Verification items for the finished model (mm, model axes). A direction names the side the tool comes from. Round coordinates to 2 decimals unless told otherwise and drop trailing zeros. Order: outer loops, then holes, each group sorted by start corner. A loop starts at its lowest first (then second) coordinate and runs counter-clockwise, first axis right, second up. Notation, with made-up numbers: M 88,-25.5 L 105,-25.5 A22 ccw 105,-4.5 Z; hole C 13.5,75.5 d10. An arc over 180 degrees is marked long. Use CSV: the item, a comma, the result in double quotes. Start each with the question number.
Q1. Sectioned sample at A-A (y = 5.1). Enter the section's corners in (x, z), and give its area (3 significant figures).
Q2. Sectioned sample at B-B (x = 8). Enter the section's corners in (y, z), and give its area (3 significant figures).
Q3. Sectioned sample at D-D (x = 61.5). Enter the section's corners in (y, z).
Q4. Gauge pin test, flat ends, axial feed: pin 1 Ø4.5 at (x, y) = (27.53, -2.9) entering from +Z; pin 2 Ø8.5 at (x, z) = (10.5, 11) entering from +Y; pin 3 Ø6 at (x, y) = (83.63, -2.9) entering from +Z; pin 4 Ø5 at (y, z) = (-3, -7) entering from -X. Record the tip position at first contact, or that the pin passes through.
Q5. Sectioned sample at C-C (y = -38.9). State how many separate pieces and enclosed holes the cut face has, and give its area (3 significant figures).
Q6. Scan lines: line 1 (X direction, y = 5, z = -23); line 2 (Y direction, x = 97.5, z = 2.5); line 3 (Z direction, x = 101.5, y = -38.9). Record each from-to range of solid material in increasing order.
Q7. Mould release check, pull along X, two halves, no side actions. Record for faces 1 (the face through (85.735, -40.244, -22.486)), 2 (the face through (0, 0, -23)), 3 (the face through (55, -42, 23.5)): +X half, -X half, draft (parallel to the pull), parting line (faces both ways), or undercut.
Q8. Set-up check for faces 4 (the face through (7.4, -27.86, 0.33)), 5 (the face through (8, -23.2, 1)), 6 (the face through (61, 41.5, 1)), 7 (the face through (100.99, -36.43, 9.46)): record each of +Z, -Z, +X, -X, +Y, -Y from which the full face is reachable in a straight line by a thin tool's end or side.
```python
from build123d import *

# Parameters (mm, degrees)
PAD_DEPTH       = 15
SKETCH001_W     = 87
SKETCH001_H     = 47
SKETCH003_W     = 87
SKETCH003_H     = 47
PAD001_DEPTH    = 82
POCKET_DEPTH    = 45
SKETCH009_R     = 2.5
POCKET001_DEPTH = 5
SKETCH010_R     = 2.5
POCKET002_DEPTH = 5


with BuildPart() as part:
    # Sketch → Pad (new body)
    with BuildSketch(Plane.YZ):
        with BuildLine():
            Line((-25.2, 23.5), (25.2, 23.5))
            ThreePointArc((25.2, -23.5), (27.86, 0), (25.2, 23.5))
            Line((25.2, -23.5), (-25.2, -23.5))
            ThreePointArc((-25.2, 23.5), (-27.86, 0), (-25.2, -23.5))
        make_face()
    extrude(amount=PAD_DEPTH)

    # Sketch002 (on Face6 of Pad) → AdditiveLoft section 0
    with BuildSketch(Plane.YZ.offset(15)):
        with BuildLine():
            Line((-25.2, 23.5), (25.2, 23.5))
            ThreePointArc((25.2, -23.5), (27.86, 0), (25.2, 23.5))
            Line((-25.2, -23.5), (25.2, -23.5))
            ThreePointArc((-25.2, 23.5), (-27.86, 0), (-25.2, -23.5))
        make_face()
    # Sketch001 → AdditiveLoft section 1
    with BuildSketch(Plane.YZ.offset(20)):
        Rectangle(SKETCH001_W, SKETCH001_H)
    loft()

    # Sketch003 (on Face10 of AdditiveLoft) → Pad001 (join)
    with BuildSketch(Plane.YZ.offset(20)):
        Rectangle(SKETCH003_W, SKETCH003_H)
    extrude(amount=PAD001_DEPTH)

    # Sketch008 (on Face10 of Pad001) → Pocket (cut)
    with BuildSketch(Plane(origin=(0, 0, 23.5), x_dir=(0, -1, 0), z_dir=(0, 0, 1))):
        Polygon((-41.5, 100), (-41.5, 21.52686), (-23.2, 16.52686), (-23.2, 0), (23.2, 0), (23.2, 16.52686), (41.5, 21.52686), (41.5, 100), align=None)
    extrude(amount=-POCKET_DEPTH, mode=Mode.SUBTRACT)

    # Sketch009 (on Face7 of Pocket) → Pocket001 (cut)
    with BuildSketch(Plane(origin=(0, 0, -21.5), x_dir=(0, -1, 0), z_dir=(0, 0, 1))):
        with Locations((-38.5, 27.52686)):
            Circle(SKETCH009_R)
        with Locations((-5.1, 27.52686)):
            Circle(SKETCH009_R)
        with Locations((-38.5, 72.72686)):
            Circle(SKETCH009_R)
        with Locations((-5.1, 72.72686)):
            Circle(SKETCH009_R)
        with Locations((2.9, 27.52686)):
            Circle(SKETCH009_R)
        with Locations((38.9, 27.52686)):
            Circle(SKETCH009_R)
        with Locations((2.9, 83.62686)):
            Circle(SKETCH009_R)
        with Locations((38.9, 83.62686)):
            Circle(SKETCH009_R)
    extrude(amount=-POCKET001_DEPTH, mode=Mode.SUBTRACT)

    # Sketch010 (on Face17 of Pocket001) → Pocket002 (cut)
    with BuildSketch(Plane(origin=(100, 0, 0), x_dir=(0, 1, 0), z_dir=(-1, 0, 0))):
        with Locations((-38.9, 7.5)):
            Circle(SKETCH010_R)
        with Locations((-38.73686, -8.5)):
            Circle(SKETCH010_R)
    extrude(amount=-POCKET002_DEPTH, mode=Mode.SUBTRACT)


solid = part.part
```
Verdict:
1,outline,"M 0,-23.5 L 25.03,-23.5 L 25.03,-21.5 L 0,-21.5 Z; M 30.03,-23.5 L 70.23,-23.5 L 70.23,-21.5 L 30.03,-21.5 Z; M 75.23,-23.5 L 102,-23.5 L 102,23.5 L 100,23.5 L 100,-21.5 L 75.23,-21.5 Z"
1,area,"274 mm²"
2,outline,"M -25.2,-23.5 L 25.2,-23.5 A105.14 ccw 25.2,23.5 L 23.2,23.5 L 23.2,-21.5 L -23.2,-21.5 L -23.2,23.5 L -25.2,23.5 A105.14 ccw Z"
2,area,"448 mm²"
3,outline,"M -43.5,-23.5 L 43.5,-23.5 L 43.5,23.5 L 41.5,23.5 L 41.5,-21.5 L -41.5,-21.5 L -41.5,23.5 L -43.5,23.5 Z"
4,pin 1,"passes through"
4,pin 2,"stops at y = 27.64"
4,pin 3,"stops at z = -21.5"
4,pin 4,"stops at x = 100"
5,separate pieces,"5"
5,enclosed holes,"0"
5,area,"316 mm²"
6,line 1,"x = 0 to 25.03, 30.02 to 70.23, 75.22 to 102"
6,line 2,"y = -43.5 to -41.5, 41.5 to 43.5"
6,line 3,"z = -23.5 to -10, -5 to 6.01, 10.99 to 23.5"
7,face 1,"undercut"
7,face 2,"-X half"
7,face 3,"draft"
8,face 4,"-X, -Y"
8,face 5,"+Z, -X"
8,face 6,"+Z"
8,face 7,"+X"
